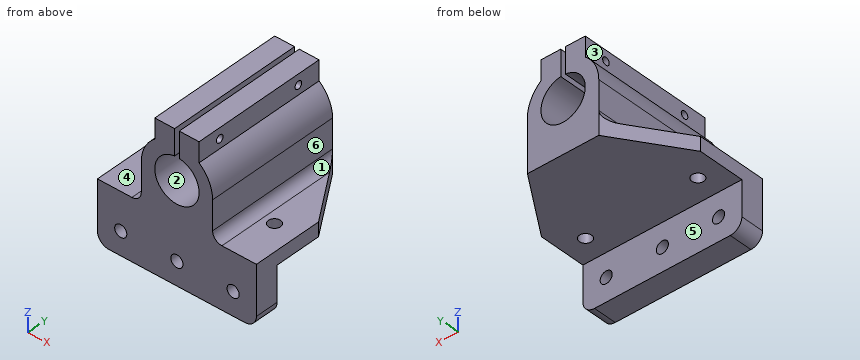
from build123d import *

# Parameters (mm, degrees)
BOSS_EXTRUDE1_DEPTH = 58
CUT_EXTRUDE1_DEPTH  = 80.848669369
SKETCH3_W           = 68.2
SKETCH3_H           = 10
BOSS_EXTRUDE2_DEPTH = 20
SKETCH4_R           = 1.6
CUT_EXTRUDE2_DEPTH  = 85.344294413
SKETCH5_R           = 2.6
CUT_EXTRUDE3_DEPTH  = 80.848669369
SKETCH6_R           = 2.6
CUT_EXTRUDE4_DEPTH  = 73.909601562
CUT_EXTRUDE5_DEPTH  = 77.784178058
FILLET1_R           = 4
FILLET2_R           = 5


with BuildPart() as part:
    # Sketch1 → Boss-Extrude1 (new body)
    with BuildSketch(Plane(origin=(0, 0, 0), x_dir=(1, 0, 0), z_dir=(0, 1, 0))):
        with BuildLine():
            Line((0, 0), (34.1, 0))
            Line((34.1, 0), (34.1, -6))
            Line((34.1, -6), (15.3, -6))
            Line((15.3, -6), (15.3, -22.5))
            ThreePointArc((15.3, -22.5), (13.77388834, -29.161080993), (9.5, -34.49333148))
            Line((9.5, -34.49333148), (9.5, -43))
            Line((9.5, -43), (-9.5, -43))
            Line((-9.5, -43), (-9.5, -34.49333148))
            ThreePointArc((-9.5, -34.49333148), (-13.77388834, -29.161080993), (-15.3, -22.5))
            Line((-15.3, -22.5), (-15.3, -6))
            Line((-15.3, -6), (-34.1, -6))
            Line((-34.1, -6), (-34.1, 0))
            Line((-34.1, 0), (0, 0))
        make_face()
    extrude(amount=BOSS_EXTRUDE1_DEPTH)

    # Sketch2 → Cut-Extrude1 (cut, through all)
    with BuildSketch(Plane(origin=(0, 58, 0), x_dir=(1, 0, 0), z_dir=(0, 1, 0))):
        with BuildLine():
            Line((-1, -31.947221814), (-1, -43))
            Line((-1, -43), (1, -43))
            Line((1, -43), (1, -31.947221814))
            ThreePointArc((1, -31.947221814), (0, -13), (-1, -31.947221814))
        make_face()
    extrude(amount=-CUT_EXTRUDE1_DEPTH, mode=Mode.SUBTRACT)

    # Sketch3 → Boss-Extrude2 (add)
    with BuildSketch(Plane(origin=(0, 0, 0), x_dir=(-1, 0, 0), z_dir=(0, 0, -1))):
        with Locations((0, 5)):
            Rectangle(SKETCH3_W, SKETCH3_H)
    extrude(amount=BOSS_EXTRUDE2_DEPTH)

    # Sketch4 → Cut-Extrude2 (cut, through all)
    with BuildSketch(Plane(origin=(9.5, 0, 0), x_dir=(0, 0, -1), z_dir=(1, 0, 0))):
        with Locations((-38.5, 48)):
            Circle(SKETCH4_R)
        with Locations((-38.5, 10)):
            Circle(SKETCH4_R)
    extrude(amount=-CUT_EXTRUDE2_DEPTH, mode=Mode.SUBTRACT)

    # Sketch5 → Cut-Extrude3 (cut, through all)
    with BuildSketch(Plane(origin=(0, 0, 0), x_dir=(-1, 0, 0), z_dir=(0, 0, -1))):
        with Locations((-24.1, 20)):
            Circle(SKETCH5_R)
        with Locations((24.1, 20)):
            Circle(SKETCH5_R)
    extrude(amount=-CUT_EXTRUDE3_DEPTH, mode=Mode.SUBTRACT)

    # Sketch6 → Cut-Extrude4 (cut, through all)
    with BuildSketch(Plane(origin=(0, 10, 0), x_dir=(1, 0, 0), z_dir=(0, 1, 0))):
        with Locations(Location((24.1, 10, 0), (0, 0, 270))):
            Circle(SKETCH6_R)
        with Locations(Location((0, 10, 0), (0, 0, 270))):
            Circle(SKETCH6_R)
        with Locations(Location((-24.1, 10, 0), (0, 0, 270))):
            Circle(SKETCH6_R)
    extrude(amount=-CUT_EXTRUDE4_DEPTH, mode=Mode.SUBTRACT)

    # Sketch7 → Cut-Extrude5 (cut, through all)
    with BuildSketch(Plane.XY.offset(6)):
        Polygon((15.3, 58), (34.1, 30), (34.1, 58), align=None)
        Polygon((-15.3, 58), (-34.1, 58), (-34.1, 30), align=None)
    extrude(amount=-CUT_EXTRUDE5_DEPTH, mode=Mode.SUBTRACT)

    # Fillet1
    fillet1_edges = [part.edges().sort_by_distance(p)[0] for p in [
        (15.3, 29, 6),
        (-15.3, 29, 6),
    ]]
    fillet(fillet1_edges, radius=FILLET1_R)

    # Fillet2
    fillet2_edges = [part.edges().sort_by_distance(p)[0] for p in [
        (-34.1, 5, -20),
        (34.1, 5, -20),
    ]]
    fillet(fillet2_edges, radius=FILLET2_R)


solid = part.part
Read the model definition and answer for the solid it produces. Units are mm, in the model's axes. Face numbers are marked on the shaded views. A direction names the side the tool comes from. Round coordinates to 2 decimals unless told otherwise and drop trailing zeros. Order: outer loops, then holes, each group sorted by start corner. A loop starts at its lowest first (then second) coordinate and runs counter-clockwise, first axis right, second up.
1) The part is cut by section C-C on x = -25. Write down the section's boundary in (y, z).
2) Flat-ended cylindrical pins translate along their axes: pin 1 (2 mm diameter, centred on x = -25.5, y = 29.5, fed in from -Z); pin 2 (16.5 mm diameter, centred on x = -28.5, y = 22, fed in from +Z); pin 3 (12 mm diameter, centred on y = 11.5, z = -3.5, fed in from +X); pin 4 (2.5 mm diameter, centred on y = 48, z = 38.5, fed in from +X). Find the tip coordinate at first contact, or state that the pin passes through.
3) The part is cut by section B-B on y = 20. Write down the section's boundary in (x, z).
4) Straight lines are drawn through the part: L1, parallel to Y at x = 3.5, z = 38.5; L2, parallel to X at y = 7, z = -10; L3, parallel to X at y = 19, z = 22. For each, find the intervals that lie inside material, in ascending order.
5) The mould has two halves that part along X. Classify the marked faces 1, 2 and 3: released by +X, released by -X, zero draft, split by the parting line, or undercut.
6) The part is cut by section A-A on z = 38.5. Write down the section's boundary in (x, y), plus the area to 3 significant figures.
7) The part is cut by section D-D on z = 26.5. Write down the section's boundary in (x, y).
8) For the marked faces 4, 5 and 6, determine the directions among +Z, -Z, +X, -X, +Y, -Y from which every point of the face is accessible in a straight line to the end or side of a thin tool.
Resolved:
1. outline: (0, -20) - (10, -20) - (10, -12.44) - (0, -12.44) - close; (0, -7.56) - (10, -7.56) - (10, 0) - (17.56, 0) - (17.56, 6) - (0, 6) - close; (22.44, 0) - (43.55, 0) - (43.55, 6) - (22.44, 6) - close
2. pin 1: stops at z = 0
2. pin 2: stops at z = 6
2. pin 3: stops at x = 34.1
2. pin 4: passes through
3. outline: (-34.1, 0) - (-26.7, 0) - (-26.7, 6) - (-34.1, 6) - close; (-21.5, 0) - (21.5, 0) - (21.5, 6) - (19.3, 6) arc R4 cw to (15.3, 10) - (15.3, 22.5) arc R15.3 ccw to (9.5, 34.49) - (9.5, 43) - (1, 43) - (1, 31.95) arc R9.5 cw (long way) to (-1, 31.95) - (-1, 43) - (-9.5, 43) - (-9.5, 34.49) arc R15.3 ccw to (-15.3, 22.5) - (-15.3, 10) arc R4 cw to (-19.3, 6) - (-21.5, 6) - close; (26.7, 0) - (34.1, 0) - (34.1, 6) - (26.7, 6) - close
4. L1: y = 0 to 8.4, 11.6 to 46.4, 49.6 to 58
4. L2: x = -34.1 to -26.7, -21.5 to -2.6, 2.6 to 21.5, 26.7 to 34.1
4. L3: x = -15.3 to -9.49, 9.49 to 15.3
5. face 1: released by +X
5. face 2: undercut
5. face 3: released by -X
6. outline: (-9.5, 0) - (-1, 0) - (-1, 8.4) - (-9.5, 8.4) - close; (-9.5, 11.6) - (-1, 11.6) - (-1, 46.4) - (-9.5, 46.4) - close; (-9.5, 49.6) - (-1, 49.6) - (-1, 58) - (-9.5, 58) - close; (1, 0) - (9.5, 0) - (9.5, 8.4) - (1, 8.4) - close; (1, 11.6) - (9.5, 11.6) - (9.5, 46.4) - (1, 46.4) - close; (1, 49.6) - (9.5, 49.6) - (9.5, 58) - (1, 58) - close
6. area: 877 mm2
7. outline: (-14.77, 0) - (-8.62, 0) - (-8.62, 58) - (-14.77, 58) - close; (8.62, 0) - (14.77, 0) - (14.77, 58) - (8.62, 58) - close
8. face 4: +Z, -X, +Y, -Y
8. face 5: -Z, +X, -X, +Y
8. face 6: +Z, +X, +Y, -Y
